Autodesk Inventor part; units mm, degrees
ref_plane "YZ Plane" through (0, 0, 0) normal (1, 0, 0) x (0, 1, 0)
ref_plane "XZ Plane" through (0, 0, 0) normal (0, 1, 0) x (-1, 0, 0)
ref_plane "XY Plane" through (0, 0, 0) normal (0, 0, 1) x (1, 0, 0)
sketch "Sketch1" plane through (0, 0, 0) normal (0, 1, 0) x (-1, 0, 0)
  line L0 (0, 0) -> (5, 0)
  line L1 (5, 0) -> (5, 9.798)
  line L2 (5, 0) -> (5, -12.702)
  line L3 (-5, -12.702) -> (-5, 9.798)
  arc A0 (5, 9.798) -> (-5, 9.798) centre (0, 0) ccw
  arc A1 (-5, -12.702) -> (5, -12.702) centre (0, 0) ccw
  dimension "d1" = 5
  dimension "d7" = 22.5
  dimension "d12" = 9.798
extrude "Extrusion1" add sketch "Sketch1" along normal blind 9
sketch "Sketch2" plane through (0, 0, 0) normal (0, -1, 0) x (1, 0, 0)
  line L0 (-5, -12.702) -> (-5, 9.798)
  line L1 (-5, -12.702) -> (-5, -1.452)
  circle A0 centre (0, -1.452) radius 2.5
  point P0 (0, 0)
  dimension "d8" = 11.25
  dimension "d9" = 5
extrude "Extrusion3" cut sketch "Sketch2" against normal blind 9
sketch "Sketch3" plane through (0, 0, 0) normal (0, -1, 0) x (1, 0, 0)
  line L0 (-5, -12.702) -> (-5, 9.798)
  line L1 (-5, 9.798) -> (-5, 12.298)
  line L2 (5, 9.798) -> (5, -12.702)
  line L3 (5, 9.798) -> (5, 12.298)
  arc A0 (5, 12.298) -> (-5, 12.298) centre (0, 2.5) ccw
  arc A1 (5, 9.798) -> (-5, 9.798) centre (0, 0) ccw
  arc A2 (5, 9.798) -> (-5, 9.798) centre (0, 0) ccw
  dimension "d13" = 2.5
  dimension "d14" = 2.5
  dimension "d15" = 11
extrude "Extrusion4" add sketch "Sketch3" against normal blind 9
properties part number "sHUFFLE"
The model under review builds one solid part; all positions refer to its coordinate system, in mm. Round coordinates to 2 decimals unless told otherwise and drop trailing zeros. Loops run counter-clockwise (first coordinate to the right, second up) from the corner with the lowest first, then second, coordinate; pieces in that order, holes last. Notation, with made-up numbers: M 77.5,6.25 L 131.5,6.25 A23 cw 131.5,23.25 Z; hole C 41,24.25 d2. An arc over 180 degrees is marked long. Put each result on its own line as item: value.
Q1. To check wall thickness, follow L1, parallel to Z at x = 0, y = 6.75; L2, parallel to X at y = 6.25, z = -3.25; L3, parallel to Z at x = -1, y = 4.5. State the ranges of each line that lie inside material, in increasing order.
Result set:
L1: z = -13.65 to -3.95, 1.05 to 13.5
L2: x = -5 to -1.74, 1.74 to 5
L3: z = -13.61 to -3.74, 0.84 to 13.45
Q2. Consider section B-B, the plane z = -3.25. Give the boundary of the cut face in (x, y).
Result set:
outline: M -5,0 L -1.74,0 L -1.74,9 L -5,9 Z; M 1.74,0 L 5,0 L 5,9 L 1.74,9 Z
Q3. Consider section C-C, the plane y = 1. Give the boundary of the cut face in (x, z), then the cut area to 3 significant figures.
Result set:
outline: M -5,-12.7 A13.65 ccw 5,-12.7 L 5,12.3 A11 ccw -5,12.3 Z; hole C 0,-1.45 d5
area: 245 mm²
Q4. Mouldability with a two-part tool opening along Z and no side actions: class faces 1 (the cylindrical face through (0.1, 4.4, 13.5)), 2 (the cylindrical face through (-0.5, 4.4, -3.9)), 3 (the flat face through (5, 4, 0)) as released by +Z, released by -Z, zero draft, split by the parting line, or undercut.
Result set:
face 1: released by +Z
face 2: undercut
face 3: zero draft
Q5. Consider section A-A, the plane x = 0. Give the boundary of the cut face in (y, z).
Result set:
outline: M 0,-13.65 L 9,-13.65 L 9,-3.95 L 0,-3.95 Z; M 0,1.05 L 9,1.05 L 9,13.5 L 0,13.5 Z
